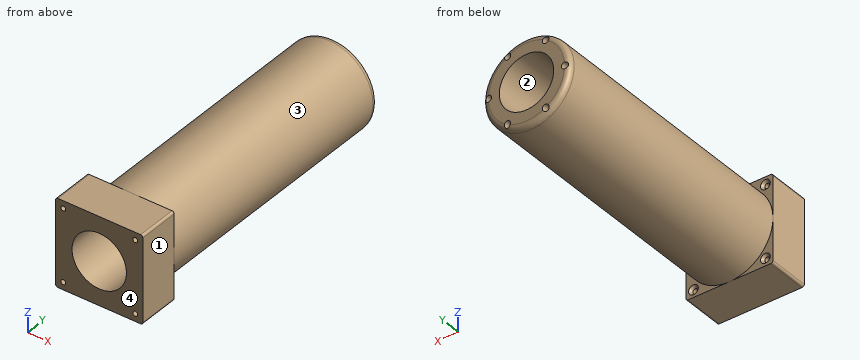
from build123d import *

# Parameters (mm, degrees)
DODANIE_WYCI_GNI_CIE1_DEPTH                        = 38
SZKIC2_R                                           = 40
DODANIE_WYCI_GNI_CIE2_DEPTH                        = 246
POG_BIENIE_STO_KOWE_POD_M4_WKR_T_Z_BEM_D           = 4.5
POG_BIENIE_STO_KOWE_POD_M4_WKR_T_Z_BEM_CSINK_D     = 8.96
POG_BIENIE_STO_KOWE_POD_M4_WKR_T_Z_BEM_CSINK_ANGLE = 90
SZKIC6_R                                           = 25
WYTNIJ_WYCI_GNI_CIE1_DEPTH                         = 290.579004764
ZAOKR_GLENIE1_R                                    = 5
OTWORY_USTALAJ_CE_6_0MM1_D                         = 6
OTWORY_USTALAJ_CE_6_0MM1_DEPTH                     = 35
OTWORY_USTALAJ_CE_6_0MM1_TIP                       = 1.802581857


with BuildPart() as part:
    # Szkic1 → Dodanie-wyciągnięcie1 (new body)
    with BuildSketch(Plane(origin=(0, 0, 0), x_dir=(1, 0, 0), z_dir=(0, 1, 0))):
        with BuildLine():
            Line((-38, -40), (38, -40))
            ThreePointArc((38, -40), (39.414213562, -39.414213562), (40, -38))
            Line((40, -38), (40, 38))
            ThreePointArc((40, 38), (39.414213562, 39.414213562), (38, 40))
            Line((38, 40), (-38, 40))
            ThreePointArc((-38, 40), (-39.414213562, 39.414213562), (-40, 38))
            Line((-40, 38), (-40, -38))
            ThreePointArc((-40, -38), (-39.414213562, -39.414213562), (-38, -40))
        make_face()
    extrude(amount=DODANIE_WYCI_GNI_CIE1_DEPTH)

    # Szkic2 → Dodanie-wyciągnięcie2 (add)
    with BuildSketch(Plane(origin=(0, 38, 0), x_dir=(1, 0, 0), z_dir=(0, 1, 0))):
        with Locations(Location((0, 0, 0), (0, 0, 270))):
            Circle(SZKIC2_R)
    extrude(amount=DODANIE_WYCI_GNI_CIE2_DEPTH)

    # Pogłębienie stożkowe pod M4 Wkręt z łbem stożkowym płaskim1 (through all)
    with Locations(Plane(origin=(0, 38, 0), x_dir=(1, 0, 0), z_dir=(0, 1, 0))):
        with Locations((-33.050252532, 33.050252532), (33.050252532, 33.050252532), (33.050252532, -33.050252532), (-33.050252532, -33.050252532)):
            CounterSinkHole(POG_BIENIE_STO_KOWE_POD_M4_WKR_T_Z_BEM_D / 2, POG_BIENIE_STO_KOWE_POD_M4_WKR_T_Z_BEM_CSINK_D / 2, counter_sink_angle=POG_BIENIE_STO_KOWE_POD_M4_WKR_T_Z_BEM_CSINK_ANGLE)

    # Szkic6 → Wytnij-wyciągnięcie1 (cut, through all)
    with BuildSketch(Plane(origin=(0, 284, 0), x_dir=(1, 0, 0), z_dir=(0, 1, 0))):
        with Locations(Location((0, 0, 0), (0, 0, 270))):
            Circle(SZKIC6_R)
    extrude(amount=-WYTNIJ_WYCI_GNI_CIE1_DEPTH, mode=Mode.SUBTRACT)

    # Zaokrąglenie1
    zaokr_glenie1_edges = [part.edges().sort_by_distance(p)[0] for p in [
        (0, 284, -40),
    ]]
    fillet(zaokr_glenie1_edges, radius=ZAOKR_GLENIE1_R)

    # Otwory ustalające Ø6.0mm1
    with Locations(Plane(origin=(0, 284, 0), x_dir=(1, 0, 0), z_dir=(0, 1, 0))):
        with Locations((-17.5, 30.310889132), (17.5, 30.310889132), (35, 0), (17.5, -30.310889132), (-17.5, -30.310889132), (-35, 0)):
            Hole(OTWORY_USTALAJ_CE_6_0MM1_D / 2, depth=OTWORY_USTALAJ_CE_6_0MM1_DEPTH)
            with Locations((0, 0, -(OTWORY_USTALAJ_CE_6_0MM1_DEPTH + OTWORY_USTALAJ_CE_6_0MM1_TIP / 2))):  # 118° drill point
                Cone(0, OTWORY_USTALAJ_CE_6_0MM1_D / 2, OTWORY_USTALAJ_CE_6_0MM1_TIP, mode=Mode.SUBTRACT)


solid = part.part
Check sheet for the modelled part. Datum: model origin and axes. Units: mm. Face numbers are marked on the shaded views. Give positions to 0.01 mm unless a question says otherwise; leave off trailing zeros. Loops run counter-clockwise (first coordinate to the right, second up) from the corner with the lowest first, then second, coordinate; pieces in that order, holes last. Notation, with made-up numbers: M -30,83.5 L 2,83.5 A20 cw 2,113.5 Z; hole C 25.25,-6 d1. An arc over 180 degrees is marked long. Return JSON: item names as keys, results as strings. Group by question number.
1. Go/stop test with flat-tipped pins: pin 1 (8 mm diameter, centred on y = 216.5, z = 10.5, fed in from +X); pin 2 (10 mm diameter, centred on y = 65, z = -29.5, fed in from +X); pin 3 (4 mm diameter, centred on y = 116, z = -32, fed in from +X). Record where each tip stops, or that it passes through.
2. Cross-section at B-B on y = 216. Record the boundary of the cut face in (x, z), plus the area to 3 significant figures.
3. Cross-section at A-A on y = 256. Record the boundary of the cut face in (x, z).
4. Mould release check, pull along X, two halves, no side actions. Record for the marked faces 1, 2, 3 and 4: released by +X, released by -X, zero draft, split by the parting line, or undercut.
5. Thickness scan on L1, parallel to Z at x = -13, y = 80; L2, parallel to Z at x = 19.5, y = 56; L3, parallel to X at y = 175, z = 0. Record the ranges inside material, lowest first.
Return value:
{
 "1": {"pin 1": "x = 39.47", "pin 2": "x = 31.62", "pin 3": "x = 26.46"},
 "2": {"outline": "C 0,0 d80; hole C 0,0 d50", "area": "3,060 mm^2"},
 "3": {"outline": "C 0,0 d80; hole C -35,0 d6; hole C 0,0 d50; hole C -17.5,-30.31 d6; hole C -17.5,30.31 d6; hole C 17.5,-30.31 d6; hole C 17.5,30.31 d6; hole C 35,0 d6"},
 "4": {"face 1": "released by +X", "face 2": "undercut", "face 3": "split by the parting line", "face 4": "zero draft"},
 "5": {"L1": "-37.83 to -21.35, 21.35 to 37.83", "L2": "-34.92 to -15.64, 15.64 to 34.92", "L3": "-40 to -25, 25 to 40"}
}
